Work out the finished part from the listing and answer in its coordinate system (mm). Face numbers are marked on the shaded views. A direction names the side the tool comes from. Round coordinates to 2 decimals unless told otherwise and drop trailing zeros. Order: outer loops, then holes, each group sorted by start corner. A loop starts at its lowest first (then second) coordinate and runs counter-clockwise, first axis right, second up. Notation, with made-up numbers: (81, -1.75) - (100, -1.75) arc R20 cw to (100, 9.25) - close; hole circle Ø1 at (14.5, -1.5). An arc over 180 degrees is marked (long way). Use CSV: the item, a comma, the result in double quotes.
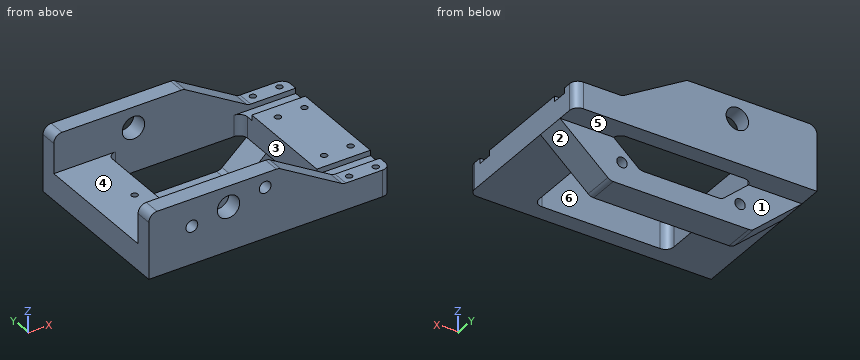
from build123d import *

# Parameters (mm, degrees)
SKETCH1_W                      = 104.14
SKETCH1_H                      = 69.85
BOSS_EXTRUDE1_DEPTH            = 23.495
SKETCH3_R                      = 4.826
PIVOT_POINTS_DEPTH             = 91.234818252
SKETCH17_W                     = 104.14
SKETCH17_H                     = 46.99
SKETCH17_H_2                   = 9.906
BOTTOM_CUTOUT_DEPTH            = 19.05
SIDE_CUTOUT_DEPTH              = 91.234818252
SKETCH20_W                     = 104.14
SKETCH20_H                     = 55.626
TOP_CUTOUT_DEPTH               = 16.51
CENTER_CUTOUT_REACH            = 71.714
SKETCH21_W                     = 58.071373626
SKETCH21_H                     = 55.626
F_8_CLEARANCE_HOLE1_D          = 4.4958
F_8_0_199_DIAMETER_HOLE1_D     = 5.0546
F_8_0_199_DIAMETER_HOLE1_DEPTH = 7.112
SKETCH30_W                     = 23.034313187
SKETCH30_H                     = 6.35
SPRING_CUTOUT_DEPTH            = 2.286
FILLET3_R                      = 3.556


# Read off the part's stored shape, not the designer's step: #6-32 Tapped Hole1
with BuildPart() as part:
    # Sketch1 → Boss-Extrude1 (new, symmetric)
    with BuildSketch(Plane.XY):
        Rectangle(SKETCH1_W, SKETCH1_H)
    extrude(amount=BOSS_EXTRUDE1_DEPTH, both=True)

    # Sketch3 → Pivot Points (cut, through all)
    with BuildSketch(Plane.XZ.offset(34.925)):
        with Locations((-17.78, 14.605)):
            Circle(SKETCH3_R)
    extrude(amount=-PIVOT_POINTS_DEPTH, mode=Mode.SUBTRACT)

    # Sketch17 → Bottom Cutout (cut)
    with BuildSketch(Plane(origin=(0, 0, -23.495), x_dir=(-1, 0, 0), z_dir=(0, 0, -1))):
        with Locations((0, -11.43)):
            Rectangle(SKETCH17_W, SKETCH17_H)
        with Locations((0, 29.972)):
            Rectangle(SKETCH17_W, SKETCH17_H_2)
    extrude(amount=-BOTTOM_CUTOUT_DEPTH, mode=Mode.SUBTRACT)

    # Sketch18 → Side Cutout (cut, through all)
    with BuildSketch(Plane.XZ.offset(34.925)):
        Polygon((52.07, 6.985), (31.75, 6.985), (3.81, 23.495), (52.07, 23.495), align=None)
        Polygon((52.07, -4.445), (30.48, -23.495), (52.07, -23.495), align=None)
        Polygon((-52.07, -4.445), (-30.48, -23.495), (-52.07, -23.495), align=None)
        Polygon((-29.035686813, -4.445), (-17.521020146, -14.605), (17.521020146, -14.605), (29.035686813, -4.445), align=None)
    extrude(amount=-SIDE_CUTOUT_DEPTH, mode=Mode.SUBTRACT)

    # Sketch20 → Top Cutout (cut)
    with BuildSketch(Plane.XY.offset(23.495)):
        Rectangle(SKETCH20_W, SKETCH20_H)
    extrude(amount=-TOP_CUTOUT_DEPTH, mode=Mode.SUBTRACT)

    # Center Cutout: up to this face of the body (flat: up to its plane)
    center_cutout_end = Plane(part.part.faces().sort_by_distance((0, -1.657135224, -4.445))[0])
    # Sketch21 → Center Cutout (cut, up to the picked face)
    with BuildSketch(Plane.XY.offset(6.985), mode=Mode.PRIVATE) as center_cutout_sk1:
        Rectangle(SKETCH21_W, SKETCH21_H)
    center_cutout_tool1 = split(extrude(center_cutout_sk1.sketch, amount=-CENTER_CUTOUT_REACH, mode=Mode.PRIVATE), bisect_by=center_cutout_end, keep=Keep.BOTH, mode=Mode.PRIVATE)
    add(center_cutout_tool1.solids().sort_by(Axis((0, 0, 6.985), (0, 0, -1)))[0], mode=Mode.SUBTRACT)

    # #8 Clearance Hole1 (through all)
    with Locations(Plane(origin=(0, 25.019, 0), x_dir=(1, 0, 0), z_dir=(0, 1, 0))):
        with Locations((25.4, 13.97), (-25.4, 13.97)):
            Hole(F_8_CLEARANCE_HOLE1_D / 2)

    # #8 (0.199) Diameter Hole1
    with Locations(Plane(origin=(0, -34.925, 0), x_dir=(-1, 0, 0), z_dir=(0, -1, 0))):
        with Locations((17.78, -14.605), (2.021106336, -17.383718139), (33.538893664, -11.826281861)):
            Hole(F_8_0_199_DIAMETER_HOLE1_D / 2, depth=F_8_0_199_DIAMETER_HOLE1_DEPTH)

    # Sketch30 → Spring Cutout (cut)
    with BuildSketch(Plane.XY.offset(6.985)):
        with Locations((40.552843407, 24.638)):
            Rectangle(SKETCH30_W, SKETCH30_H)
        with Locations((40.552843407, -24.638)):
            Rectangle(SKETCH30_W, SKETCH30_H)
    extrude(amount=-SPRING_CUTOUT_DEPTH, mode=Mode.SUBTRACT)

    # #6-32 Tapped Hole1 outline → #6-32 Tapped Hole1 (revolve, cut)
    with BuildSketch(Plane(origin=(36.195, -31.75, 0), x_dir=(1, 0, 0), z_dir=(0, -1, 0))):
        Polygon((0, 6.985), (0, -3.22569403), (1.35255, -2.413), (1.35255, 6.985), align=None)
    revolve(axis=Axis((36.195, -31.75, 0), (0, 0, 1)), mode=Mode.SUBTRACT)

    # 6-32 Tapped Hole1 2 outline → 6-32 Tapped Hole1 2 (revolve, cut)
    with BuildSketch(Plane(origin=(36.195, -15.24, 0), x_dir=(1, 0, 0), z_dir=(0, -1, 0))):
        Polygon((0, 6.985), (0, -3.22569403), (1.35255, -2.413), (1.35255, 6.985), align=None)
    revolve(axis=Axis((36.195, -15.24, 0), (0, 0, 1)), mode=Mode.SUBTRACT)

    # 6-32 Tapped Hole1 3 outline → 6-32 Tapped Hole1 3 (revolve, cut)
    with BuildSketch(Plane(origin=(47.625, -15.24, 0), x_dir=(1, 0, 0), z_dir=(0, -1, 0))):
        Polygon((0, 6.985), (0, -3.22569403), (1.35255, -2.413), (1.35255, 6.985), align=None)
    revolve(axis=Axis((47.625, -15.24, 0), (0, 0, 1)), mode=Mode.SUBTRACT)

    # 6-32 Tapped Hole1 4 outline → 6-32 Tapped Hole1 4 (revolve, cut)
    with BuildSketch(Plane(origin=(47.625, -31.75, 0), x_dir=(1, 0, 0), z_dir=(0, -1, 0))):
        Polygon((0, 6.985), (0, -3.22569403), (1.35255, -2.413), (1.35255, 6.985), align=None)
    revolve(axis=Axis((47.625, -31.75, 0), (0, 0, 1)), mode=Mode.SUBTRACT)

    # 6-32 Tapped Hole1 5 outline → 6-32 Tapped Hole1 5 (revolve, cut)
    with BuildSketch(Plane(origin=(47.625, 31.75, 0), x_dir=(1, 0, 0), z_dir=(0, -1, 0))):
        Polygon((0, 6.985), (0, -3.22569403), (1.35255, -2.413), (1.35255, 6.985), align=None)
    revolve(axis=Axis((47.625, 31.75, 0), (0, 0, 1)), mode=Mode.SUBTRACT)

    # 6-32 Tapped Hole1 6 outline → 6-32 Tapped Hole1 6 (revolve, cut)
    with BuildSketch(Plane(origin=(36.195, 15.24, 0), x_dir=(1, 0, 0), z_dir=(0, -1, 0))):
        Polygon((0, 6.985), (0, -3.22569403), (1.35255, -2.413), (1.35255, 6.985), align=None)
    revolve(axis=Axis((36.195, 15.24, 0), (0, 0, 1)), mode=Mode.SUBTRACT)

    # 6-32 Tapped Hole1 7 outline → 6-32 Tapped Hole1 7 (revolve, cut)
    with BuildSketch(Plane(origin=(47.625, 15.24, 0), x_dir=(1, 0, 0), z_dir=(0, -1, 0))):
        Polygon((0, 6.985), (0, -3.22569403), (1.35255, -2.413), (1.35255, 6.985), align=None)
    revolve(axis=Axis((47.625, 15.24, 0), (0, 0, 1)), mode=Mode.SUBTRACT)

    # 6-32 Tapped Hole1 8 outline → 6-32 Tapped Hole1 8 (revolve, cut)
    with BuildSketch(Plane(origin=(36.195, 31.75, 0), x_dir=(1, 0, 0), z_dir=(0, -1, 0))):
        Polygon((0, 6.985), (0, -3.22569403), (1.35255, -2.413), (1.35255, 6.985), align=None)
    revolve(axis=Axis((36.195, 31.75, 0), (0, 0, 1)), mode=Mode.SUBTRACT)

    # 6-32 Tapped Hole1 9 outline → 6-32 Tapped Hole1 9 (revolve, cut)
    with BuildSketch(Plane(origin=(-35.385686813, 0, 0), x_dir=(1, 0, 0), z_dir=(0, -1, 0))):
        Polygon((0, 6.985), (0, -3.22569403), (1.35255, -2.413), (1.35255, 6.985), align=None)
    revolve(axis=Axis((-35.385686813, 0, 0), (0, 0, 1)), mode=Mode.SUBTRACT)

    # Fillet3
    # the kernel refuses this fillet: 3.556 mm, written as the material it adds along each edge
    with BuildSketch(Plane(origin=(31.75, -34.925, 6.985), x_dir=(1, 0, 0), z_dir=(0, 1, 0)), Plane(origin=(31.75, 27.813, 6.985), x_dir=(1, 0, 0), z_dir=(0, 1, 0))) as fillet3_piece_1:
        with BuildLine():
            CenterArc((FILLET3_R * 0.273374206028, -FILLET3_R), FILLET3_R, 90, 30.579226872)
            Line((-FILLET3_R * 0.235355106099, -FILLET3_R * 0.139073471786), (0, 0))
            Line((0, 0), (FILLET3_R * 0.273374206028, 0))
        make_face()
    extrude(amount=7.112)
    with BuildSketch(Plane(origin=(29.035686813, -27.813, 4.699), x_dir=(-1, 0, 0), z_dir=(0, 0, -1))) as fillet3_piece_2:
        with BuildLine():
            CenterArc((FILLET3_R, FILLET3_R), FILLET3_R, 180, 90)
            Line((0, FILLET3_R), (0, 0))
            Line((0, 0), (FILLET3_R, 0))
        make_face()
    extrude(amount=9.144)
    with BuildSketch(Plane(origin=(29.035686813, 27.813, 4.699), x_dir=(-1, 0, 0), z_dir=(0, 0, -1))) as fillet3_piece_3:
        with BuildLine():
            CenterArc((FILLET3_R, -FILLET3_R), FILLET3_R, 90, 90)
            Line((0, -FILLET3_R), (0, 0))
            Line((0, 0), (FILLET3_R, 0))
        make_face()
    extrude(amount=9.144)
    with BuildSketch(Plane(origin=(29.035686813, 27.813, 4.699), x_dir=(-1, 0, 0), z_dir=(0, 0, -1))) as fillet3_piece_4_section:
        with BuildLine():
            CenterArc((FILLET3_R, -FILLET3_R), FILLET3_R, 90, 90)
            Line((0, -FILLET3_R), (0, 0))
            Line((0, 0), (FILLET3_R, 0))
        make_face()
    fillet3_piece_4 = extrude(amount=18.034, mode=Mode.PRIVATE)
    fillet3_piece_4 = split(fillet3_piece_4, bisect_by=Plane(origin=(28.996396746, 25.019, -4.462333853), z_dir=(0, -1, 0)), keep=Keep.TOP, mode=Mode.PRIVATE)
    add(fillet3_piece_4)
    with BuildSketch(Plane(origin=(-29.035686813, 27.813, 6.985), x_dir=(1, 0, 0), z_dir=(0, 0, -1))) as fillet3_piece_5:
        with BuildLine():
            CenterArc((FILLET3_R, FILLET3_R), FILLET3_R, 180, 90)
            Line((0, FILLET3_R), (0, 0))
            Line((0, 0), (FILLET3_R, 0))
        make_face()
    extrude(amount=11.43)
    with BuildSketch(Plane(origin=(-29.035686813, 27.813, 6.985), x_dir=(1, 0, 0), z_dir=(0, 0, -1))) as fillet3_piece_6_section:
        with BuildLine():
            CenterArc((FILLET3_R, FILLET3_R), FILLET3_R, 180, 90)
            Line((0, FILLET3_R), (0, 0))
            Line((0, 0), (FILLET3_R, 0))
        make_face()
    fillet3_piece_6 = extrude(amount=20.32, mode=Mode.PRIVATE)
    fillet3_piece_6 = split(fillet3_piece_6, bisect_by=Plane(origin=(-28.996396746, 25.019, -4.462333853), z_dir=(0, -1, 0)), keep=Keep.TOP, mode=Mode.PRIVATE)
    add(fillet3_piece_6)
    with BuildSketch(Plane(origin=(-29.035686813, -27.813, 6.985), x_dir=(1, 0, 0), z_dir=(0, 0, -1))) as fillet3_piece_7:
        with BuildLine():
            CenterArc((FILLET3_R, -FILLET3_R), FILLET3_R, 90, 90)
            Line((0, -FILLET3_R), (0, 0))
            Line((0, 0), (FILLET3_R, 0))
        make_face()
    extrude(amount=11.43)
    with BuildSketch(Plane(origin=(17.521020146, 12.065, -14.605), x_dir=(-1, 0, 0), z_dir=(0, 1, 0)), Plane(origin=(-17.521020146, 12.065, -14.605), x_dir=(-0.7498378553650912, 0, 0.6616216370868477), z_dir=(0, 1, 0))) as fillet3_piece_8:
        with BuildLine():
            CenterArc((FILLET3_R * 0.378104539834, FILLET3_R), FILLET3_R, 228.576334375, 41.423665625)
            Line((-FILLET3_R * 0.283517097253, FILLET3_R * 0.250162144635), (0, 0))
            Line((0, 0), (FILLET3_R * 0.378104539834, 0))
        make_face()
    extrude(amount=12.954)
    # the kernel refuses this fillet: 3.556 mm, written as the material it takes off along each edge
    with BuildSketch(Plane(origin=(3.81, -37.355296692, 23.495), x_dir=(-1, 0, 0), z_dir=(0, 1, 0))) as fillet3_2_piece_1:
        with BuildLine():
            CenterArc((FILLET3_R * 0.273374206028, -FILLET3_R), FILLET3_R, 90, 30.579226872)
            Line((-FILLET3_R * 0.235355106099, -FILLET3_R * 0.139073471786), (0, 0))
            Line((0, 0), (FILLET3_R * 0.273374206028, 0))
        make_face()
    extrude(amount=11.972593383, mode=Mode.SUBTRACT)
    with BuildSketch(Plane(origin=(-52.07, -18.923, 23.495), x_dir=(1, 0, 0), z_dir=(0, -1, 0)), Plane(origin=(-52.07, 43.815, 23.495), x_dir=(1, 0, 0), z_dir=(0, -1, 0))) as fillet3_2_piece_2:
        with BuildLine():
            CenterArc((FILLET3_R, -FILLET3_R), FILLET3_R, 90, 90)
            Line((0, -FILLET3_R), (0, 0))
            Line((0, 0), (FILLET3_R, 0))
        make_face()
    extrude(amount=24.892, mode=Mode.SUBTRACT)
    with BuildSketch(Plane(origin=(52.07, 34.925, 15.875), x_dir=(-1, 0, 0), z_dir=(0, 0, -1))) as fillet3_2_piece_3:
        with BuildLine():
            CenterArc((FILLET3_R, -FILLET3_R), FILLET3_R, 90, 90)
            Line((0, -FILLET3_R), (0, 0))
            Line((0, 0), (FILLET3_R, 0))
        make_face()
    extrude(amount=29.21, mode=Mode.SUBTRACT)
    with BuildSketch(Plane(origin=(52.07, -34.925, 15.875), x_dir=(-1, 0, 0), z_dir=(0, 0, -1))) as fillet3_2_piece_4:
        with BuildLine():
            CenterArc((FILLET3_R, FILLET3_R), FILLET3_R, 180, 90)
            Line((0, FILLET3_R), (0, 0))
            Line((0, 0), (FILLET3_R, 0))
        make_face()
    extrude(amount=29.21, mode=Mode.SUBTRACT)
    with BuildSketch(Plane(origin=(3.81, 25.382703308, 23.495), x_dir=(0.8609265282143158, 0, -0.5087293121266405), z_dir=(0, 1, 0))) as fillet3_2_piece_5:
        with BuildLine():
            CenterArc((FILLET3_R * 0.273374206028, FILLET3_R), FILLET3_R, 239.420773128, 30.579226872)
            Line((-FILLET3_R * 0.235355106099, FILLET3_R * 0.139073471786), (0, 0))
            Line((0, 0), (FILLET3_R * 0.273374206028, 0))
        make_face()
    extrude(amount=11.972593383, mode=Mode.SUBTRACT)
    with BuildSketch(Plane(origin=(-30.48, 8.703650641, -23.495), x_dir=(-0.7498378553650943, 0, 0.6616216370868445), z_dir=(0, 1, 0))) as fillet3_2_piece_6:
        with BuildLine():
            CenterArc((FILLET3_R * 0.378104539834, FILLET3_R), FILLET3_R, 228.576334375, 41.423665625)
            Line((-FILLET3_R * 0.283517097253, FILLET3_R * 0.250162144635), (0, 0))
            Line((0, 0), (FILLET3_R * 0.378104539834, 0))
        make_face()
    extrude(amount=19.676698718, mode=Mode.SUBTRACT)
    with BuildSketch(Plane(origin=(30.48, 8.703650641, -23.495), x_dir=(0.7498378553650921, 0, 0.6616216370868468), z_dir=(0, 1, 0))) as fillet3_2_piece_7:
        with BuildLine():
            CenterArc((FILLET3_R * 0.378104539834, -FILLET3_R), FILLET3_R, 90, 41.423665625)
            Line((-FILLET3_R * 0.283517097253, -FILLET3_R * 0.250162144635), (0, 0))
            Line((0, 0), (FILLET3_R * 0.378104539834, 0))
        make_face()
    extrude(amount=19.676698718, mode=Mode.SUBTRACT)


solid = part.part
(1) Find section A-A (y = 4.5). Determine the outline of the cut face in (x, z) (3 decimals).
Findings below:
outline,"(-52.07, -4.445) - (-29.036, -4.445) - (-29.036, 6.985) - (-52.07, 6.985) - close; (29.036, -4.445) - (52.07, -4.445) - (52.07, 6.985) - (29.036, 6.985) - close"
(2) Find the intervals of material crossed by L1, parallel to Y at x = -1, z = -3 (3 decimals); L2, parallel to X at y = 17, z = -13; L3, parallel to Y at x = 37, z = -2.5 (3 decimals), in increasing order. Write a range as from..to.
Findings below:
L1,"y = -34.925..-27.813, 27.813..34.925"
L2,"x = -42.37..-27.43, -23.37..-19.34, 19.34..23.37, 27.43..42.37"
L3,"y = -34.925..-32.65, -30.85..-16.14, -14.34..14.34, 16.14..30.85, 32.65..34.925"
(3) Find section C-C (x = -42). Determine the outline of the cut face in (y, z) (3 decimals).
Findings below:
outline,"(-34.925, -4.445) - (12.065, -4.445) - (12.065, -13.33) - (25.019, -13.33) - (25.019, -4.445) - (34.925, -4.445) - (34.925, 23.495) - (27.813, 23.495) - (27.813, 6.985) - (-27.813, 6.985) - (-27.813, 23.495) - (-34.925, 23.495) - close"
(4) Each of these flat-tipped pins is pushed along its axis until it touches: pin 1 (4 mm diameter, centred on x = -9.5, z = -17.5, fed in from +Y); pin 2 (4 mm diameter, centred on x = -33.54, z = 11.83, fed in from -Y); pin 3 (1.5 mm diameter, centred on x = 34.5, y = 15, fed in from -Z); pin 4 (8.5 mm diameter, centred on x = -17.78, z = 14.605, fed in from -Y). Where does it stop, or does it pass through?
Findings below:
pin 1,"stops at y = 25.02"
pin 2,"stops at y = 27.81"
pin 3,"stops at z = -20.61"
pin 4,"passes through"
(5) For the marked faces 4, 5 and 6, determine the directions among +Z, -Z, +X, -X, +Y, -Y from which every point of the face is accessible in a straight line to the end or side of a thin tool.
Findings below:
face 4,"+Z, +X, -X"
face 5,"-Z, +X, -X, +Y"
face 6,"+Z"
(6) Find section D-D (z = -17.5). Determine the outline of the cut face in (x, y) (3 decimals).
Findings below:
outline,"(-37.274, 12.065) - (37.274, 12.065) - (37.274, 25.019) - (-37.274, 25.019) - close"
(7) The mould has two halves that part along Y. Classify the marked faces 1, 2 and 3: released by +Y, released by -Y, zero draft, split by the parting line, or undercut.
Findings below:
face 1,"released by +Y"
face 2,"zero draft"
face 3,"undercut"
(8) Find section B-B (z = -6). Determine the outline of the cut face in (x, y) (3 decimals).
Findings below:
outline,"(-50.308, 12.065) - (-27.273, 12.065) - (-27.273, 25.019) - (-50.308, 25.019) - close; (27.273, 12.065) - (50.308, 12.065) - (50.308, 25.019) - (27.273, 25.019) - close"
